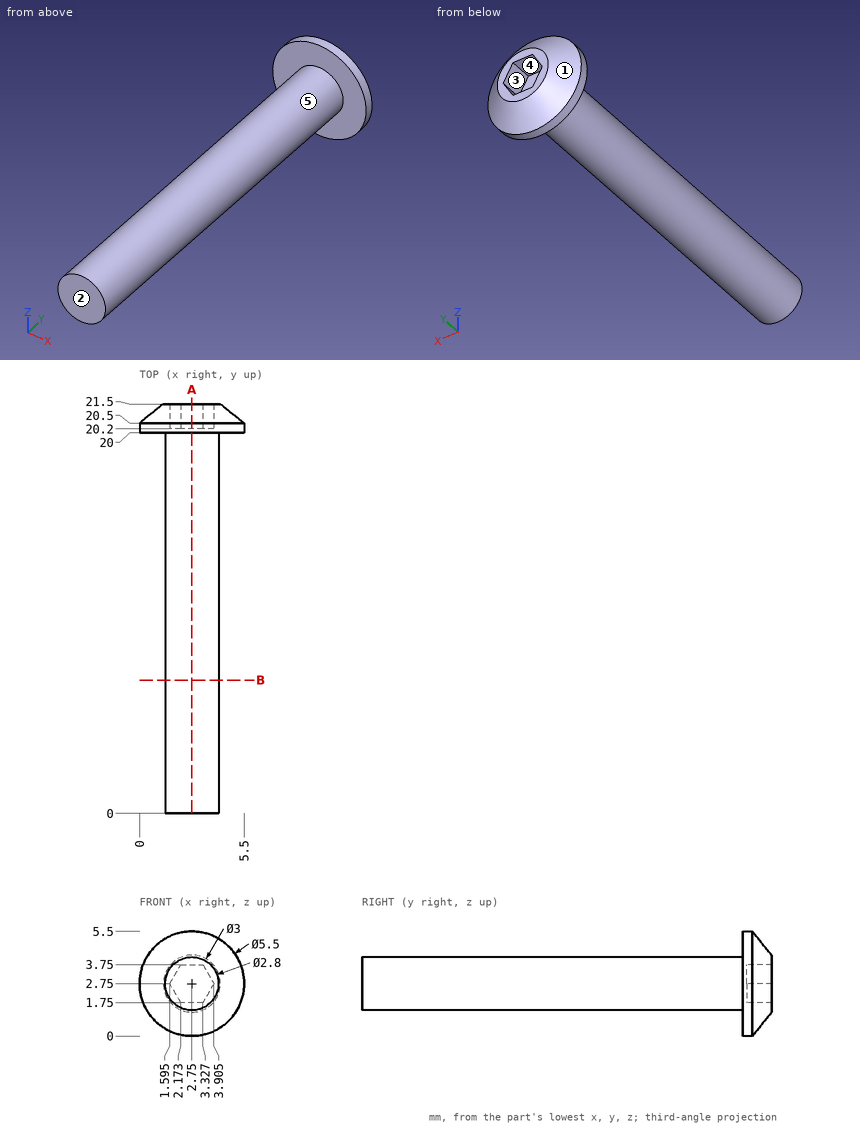
Geometry: see drawing. Coordinates: mm, zero at the bounding-box minimum. A direction names the side the tool comes from. Coordinates: 2 decimals unless noted, no trailing zeros. Loops run counter-clockwise (first coordinate to the right, second up) from the corner with the lowest first, then second, coordinate; pieces in that order, holes last. Notation, with made-up numbers: M 80,-10.75 L 122,-10.75 A11 ccw 122,-4.75 Z; hole C 7.25,29.25 d10. An arc over 180 degrees is marked long. Put each result on its own line as item: value. Start each with the question number.
1) Cut plane A-A on x = 2.75. Return the cut outline in (y, z).
2) Pull-direction query (Z, two-part tool) for the marked faces 1, 2 and 3; classes: pulls with the +Z half, pulls with the -Z half, needs draft (parallel to the pull), parting line crosses it, or undercut.
3) Ray query, L1, parallel to Y at x = 2.5, z = 3.6; L2, parallel to Y at x = 3.1, z = 1.25; L3, parallel to Z at x = 3.05, y = 18.5. Return the intervals inside material, ascending. Write a range as from..to.
4) Reachability of the marked faces 4 and 5 from +Z, -Z, +X, -X, +Y, -Y: full face, straight path, thin tool, end or side. Return the list, or none.
5) Cut plane B-B on y = 7. Return the cut outline in (x, z).
6) Contact query for flat-ended pins moving along their axis: pin 1 Ø1 at (y, z) = (14, 2) entering from +X; pin 2 Ø1.6 at (x, z) = (3, 2.5) entering from +Y; pin 3 Ø1.5 at (x, y) = (1.5, 15.5) entering from -Z. Output: stop coordinate, or through.
The answers:
1. outline: M 0,1.35 L 20,1.35 L 20,0 L 20.5,0 L 21.5,1.25 L 21.5,1.75 L 20.2,1.75 L 20.2,3.75 L 21.5,3.75 L 21.5,4.25 L 20.5,5.5 L 20,5.5 L 20,4.15 L 0,4.15 Z
2. face 1: parting line crosses it
2. face 2: needs draft
2. face 3: undercut
3. L1: y = 0..20.2
3. L2: y = 20..21.47
3. L3: z = 1.38..4.12
4. face 4: +Y
4. face 5: -Y
5. outline: C 2.75,2.75 d2.8
6. pin 1: stops at x = 4.13
6. pin 2: stops at y = 21.5
6. pin 3: stops at z = 1.44
